```python
from build123d import *

# Parameters (mm, degrees)
SKETCH_1_R             = 10
SM_BASE_FLANGE_1_DEPTH = 3
SKETCH_6_R             = 5.25
CUT_EXTRUDE_1_DEPTH    = 2
SKETCH_7_R             = 1
CUT_EXTRUDE_2_DEPTH    = 15.456832295


# Sheet-metal steps are written as plain solids
with BuildPart() as part:
    # Sketch 1 → 基体-法兰1 (new body)
    with BuildSketch(Plane(origin=(0, 0, 0), x_dir=(1, 0, 0), z_dir=(0, 1, 0))):
        with Locations(Location((0, 0, 0), (0, 0, 270))):
            Circle(SKETCH_1_R)
    extrude(amount=-SM_BASE_FLANGE_1_DEPTH)

    # 草图6 → 切除-拉伸1 (cut)
    with BuildSketch(Plane(origin=(0, 0, 0), x_dir=(1, 0, 0), z_dir=(0, 1, 0))):
        with Locations(Location((0, 0, 0), (0, 0, 270))):
            Circle(SKETCH_6_R)
    extrude(amount=-CUT_EXTRUDE_1_DEPTH, mode=Mode.SUBTRACT)

    # 草图7 → 切除-拉伸2 (cut, through all)
    with BuildSketch(Plane(origin=(0, 0, 0), x_dir=(1, 0, 0), z_dir=(0, 1, 0))):
        with Locations(Location((0, 8, 0), (0, 0, 270))):
            Circle(SKETCH_7_R)
        with Locations(Location((5.656854249, 5.656854249, 0), (0, 0, 270))):
            Circle(SKETCH_7_R)
        with Locations(Location((8, 0, 0), (0, 0, 270))):
            Circle(SKETCH_7_R)
        with Locations(Location((5.656854249, -5.656854249, 0), (0, 0, 270))):
            Circle(SKETCH_7_R)
        with Locations(Location((0, -8, 0), (0, 0, 270))):
            Circle(SKETCH_7_R)
        with Locations(Location((-5.656854249, -5.656854249, 0), (0, 0, 270))):
            Circle(SKETCH_7_R)
        with Locations(Location((-8, 0, 0), (0, 0, 270))):
            Circle(SKETCH_7_R)
        with Locations(Location((-5.656854249, 5.656854249, 0), (0, 0, 270))):
            Circle(SKETCH_7_R)
    extrude(amount=-CUT_EXTRUDE_2_DEPTH, mode=Mode.SUBTRACT)


solid = part.part
```
Source: CAD feature listing. Evaluate the final solid. Frame: model axes, mm. A direction names the side the tool comes from. Coordinates: 2 decimals unless noted, no trailing zeros. Loops run counter-clockwise (first coordinate to the right, second up) from the corner with the lowest first, then second, coordinate; pieces in that order, holes last. Notation, with made-up numbers: M 22.25,-18 L 60.25,-18 A29 cw 60.25,10 Z; hole C 29,-6 d2. An arc over 180 degrees is marked long. Use CSV: the item, a comma, the result in double quotes.
(1) Cut plane B-B on x = 0. Return loops of the section in (y, z), and give its area (3 significant figures).
Answers follow:
outline,"M -3,-10 L 0,-10 L 0,-9 L -3,-9 Z; M -3,-7 L 0,-7 L 0,-5.25 L -2,-5.25 L -2,5.25 L 0,5.25 L 0,7 L -3,7 Z; M -3,9 L 0,9 L 0,10 L -3,10 Z"
area,"27.0 mm²"
(2) Contact query for flat-ended pins moving along their axis: pin 1 (2.5 mm diameter, centred on x = -5.66, z = 5.66, fed in from -Y); pin 2 (1.6 mm diameter, centred on x = 5.66, z = -5.66, fed in from +Y); pin 3 (1 mm diameter, centred on y = -2, z = 7, fed in from +X); pin 4 (1.5 mm diameter, centred on x = 2.5, y = -2, fed in from -Z). Output: stop coordinate, or through.
Answers follow:
pin 1,"y = -3"
pin 2,"through"
pin 3,"x = 7.6"
pin 4,"z = -9.85"
(3) Cut plane A-A on z = 0. Return loops of the section in (x, y).
Answers follow:
outline,"M -10,-3 L -9,-3 L -9,0 L -10,0 Z; M -7,-3 L 7,-3 L 7,0 L 5.25,0 L 5.25,-2 L -5.25,-2 L -5.25,0 L -7,0 Z; M 9,-3 L 10,-3 L 10,0 L 9,0 Z"
(4) Cut plane C-C on z = 8. Return loops of the section in (x, y), and give its area (3 significant figures).
Answers follow:
outline,"M -6,-3 L -1,-3 L -1,0 L -6,0 Z; M 1,-3 L 6,-3 L 6,0 L 1,0 Z"
area,"30.0 mm²"
(5) Line query: line 1 (X direction, y = -1.6, z = 0); line 2 (X direction, y = -0.65, z = -4.75); line 3 (Z direction, x = -5.5, y = -2.2). Output: solid intervals per line, ascending. Write a range as [from, to].
Answers follow:
line 1,"[-10, -9], [-7, -5.25], [5.25, 7], [9, 10]"
line 2,"[-8.8, -6.08], [-5.24, -2.24], [2.24, 5.24], [6.08, 8.8]"
line 3,"[-8.35, -6.64], [-4.67, 4.67], [6.64, 8.35]"
(6) Cut plane D-D on x = 8.25. Return loops of the section in (y, z), and give its area (3 significant figures).
Answers follow:
outline,"M -3,-5.65 L 0,-5.65 L 0,-0.97 L -3,-0.97 Z; M -3,0.97 L 0,0.97 L 0,5.65 L -3,5.65 Z"
area,"28.1 mm²"
(7) Draft query along X for faces 1 (the face through (-4, 0, 4)), 2 (the face through (-1, -1, 8)), 3 (the face through (-9.76, -1.48, -2.17)). Return one class per face: pulls with the +X half, pulls with the -X half, needs draft (parallel to the pull), parting line crosses it, or undercut.
Answers follow:
face 1,"needs draft"
face 2,"undercut"
face 3,"parting line crosses it"
(8) Reachability of faces 4 (the face through (0, -3, 0)), 5 (the face through (0, -2, 0)) from +Z, -Z, +X, -X, +Y, -Y: full face, straight path, thin tool, end or side. Return the list, or none.
Answers follow:
face 4,"+Z, -Z, +X, -X, -Y"
face 5,"+Y"
